Geometry: final body of the model. Coordinates: model frame, mm. Face numbers are marked on the shaded views. A direction names the side the tool comes from. Give positions to 0.01 mm unless a question says otherwise; leave off trailing zeros. Loops run counter-clockwise (first coordinate to the right, second up) from the corner with the lowest first, then second, coordinate; pieces in that order, holes last.
1. Access query for the marked faces 1 and 2. Directions: +Z, -Z, +X, -X, +Y, -Y. A direction counts if a zero-diameter tool reaches every point of the face in a straight line with its end or side. Return the directions, or none.
2. Section D-D, the plane z = -57.5. Output: boundary loops of the cut face in (x, y), then the cut area to 3 significant figures.
3. Material intervals for line 1 along Y through (x, z) = (2.25, -9); line 2 along Y through (x, z) = (2.25, -50); line 3 along Z through (x, y) = (2, 41.25), sorted ascending.
4. First-contact query: P1, Ø0.9, axis at x = 4.5, z = -26, coming from the +Y side; P2, Ø4, axis at y = 47, z = -23, coming from the -X side; P3, Ø6.5, axis at y = 47.5, z = -29.5, coming from the +X side; P4, Ø1.8, axis at y = 47, z = -37, coming from the +X side. Flat tips, straight axial feed; report the tip coordinate or a pass-through.
5. Section C-C, the plane z = -50. Output: boundary loops of the cut face in (x, y), then the cut area to 3 significant figures.
6. Section B-B, the plane y = 42. Output: boundary loops of the cut face in (x, z), then the cut area to 3 significant figures.
from build123d import *

# Parameters (mm, degrees)
SKETCH27_R          = 4
SKETCH27_R_2        = 2.5
BOSS_EXTRUDE1_DEPTH = 6
SKETCH33_R          = 4.99
CUT_EXTRUDE2_DEPTH  = 3
SKETCH34_W          = 20
SKETCH34_H          = 6
CUT_EXTRUDE3_DEPTH  = 3
CUT_EXTRUDE5_REACH  = 84.855
SKETCH36_R          = 1.5
FILLET3_R           = 2
FILLET4_R           = 10
CUT_EXTRUDE6_REACH  = 85.018
CHAMFER1_SIZE       = 1.5


with BuildPart() as part:
    # Sketch27 → Boss-Extrude1 (new body)
    with BuildSketch(Plane(origin=(0, 0, 0), x_dir=(0, 0, -1), z_dir=(1, 0, 0))):
        with BuildLine():
            Line((9, 50), (66, 50))
            Line((66, 50), (66, 45))
            Line((66, 45), (48.564398788, 34))
            Line((48.564398788, 34), (9, 34))
            ThreePointArc((9, 34), (1, 42), (9, 50))
        make_face()
        with Locations((9, 42)):
            Circle(SKETCH27_R, mode=Mode.SUBTRACT)
        with Locations((50, 42)):
            Circle(SKETCH27_R_2, mode=Mode.SUBTRACT)
    extrude(amount=BOSS_EXTRUDE1_DEPTH)

    # Sketch33 → Cut-Extrude2 (cut)
    with BuildSketch(Plane(origin=(6, 0, 0), x_dir=(0, 0, -1), z_dir=(1, 0, 0))):
        with Locations((9, 42)):
            Circle(SKETCH33_R)
    extrude(amount=-CUT_EXTRUDE2_DEPTH, mode=Mode.SUBTRACT)

    # Sketch34 → Cut-Extrude3 (cut)
    with BuildSketch(Plane(origin=(6, 0, 0), x_dir=(0, 0, -1), z_dir=(1, 0, 0))):
        with Locations((30, 47)):
            Rectangle(SKETCH34_W, SKETCH34_H)
    extrude(amount=-CUT_EXTRUDE3_DEPTH, mode=Mode.SUBTRACT)

    # Sketch36 → Cut-Extrude5 (cut, up to next)
    with BuildSketch(Plane(origin=(3, 0, 0), x_dir=(0, 0, -1), z_dir=(1, 0, 0)), mode=Mode.PRIVATE) as cut_extrude5_sk1:
        with Locations((23, 47)):
            Circle(SKETCH36_R)
    cut_extrude5_tool1 = extrude(cut_extrude5_sk1.sketch, amount=-CUT_EXTRUDE5_REACH, mode=Mode.PRIVATE) & part.part
    # Sketch36 → Cut-Extrude5 (cut, up to next)
    with BuildSketch(Plane(origin=(3, 0, 0), x_dir=(0, 0, -1), z_dir=(1, 0, 0)), mode=Mode.PRIVATE) as cut_extrude5_sk2:
        with Locations((37, 47)):
            Circle(SKETCH36_R)
    cut_extrude5_tool2 = extrude(cut_extrude5_sk2.sketch, amount=-CUT_EXTRUDE5_REACH, mode=Mode.PRIVATE) & part.part
    add(cut_extrude5_tool1.solids().sort_by_distance((3, 47, -23))[0], mode=Mode.SUBTRACT)
    add(cut_extrude5_tool2.solids().sort_by_distance((3, 47, -37))[0], mode=Mode.SUBTRACT)

    # Fillet3
    fillet3_edges = [part.edges().sort_by_distance(p)[0] for p in [
        (3, 50, -66),
        (3, 45, -66),
    ]]
    fillet(fillet3_edges, radius=FILLET3_R)

    # Fillet4
    fillet4_edges = [part.edges().sort_by_distance(p)[0] for p in [
        (3, 34, -48.564398788),
    ]]
    fillet(fillet4_edges, radius=FILLET4_R)

    # Sketch37 → Cut-Extrude6 (cut, up to next)
    with BuildSketch(Plane(origin=(6, 0, 0), x_dir=(0, 0, -1), z_dir=(1, 0, 0)), mode=Mode.PRIVATE) as cut_extrude6_sk1:
        with BuildLine():
            Line((20.313708499, 38), (42.254033308, 38))
            ThreePointArc((42.254033308, 38), (44.754033308, 37.682458366), (47.09526249, 36.75))
            ThreePointArc((47.09526249, 36.75), (50.17237218, 36.002476525), (53.201469536, 36.925495807))
            Line((53.201469536, 36.925495807), (53.201469536, 34))
            Line((53.201469536, 34), (9, 34))
            ThreePointArc((9, 34), (11.666666667, 34.457527667), (14.028314888, 35.777777778))
            ThreePointArc((14.028314888, 35.777777778), (16.980375166, 37.428090416), (20.313708499, 38))
        make_face()
    cut_extrude6_tool1 = extrude(cut_extrude6_sk1.sketch, amount=-CUT_EXTRUDE6_REACH, mode=Mode.PRIVATE) & part.part
    add(cut_extrude6_tool1.solids().sort_by_distance((6, 35.823598, -32.372789))[0], mode=Mode.SUBTRACT)

    # Chamfer1
    chamfer1_edges = [part.edges().sort_by_distance(p)[0] for p in [
        (0, 47, -21.5),
        (0, 47, -35.5),
    ]]
    chamfer(chamfer1_edges, length=CHAMFER1_SIZE - 0.0001)  # a hair under: the kernel refuses the full size


solid = part.part
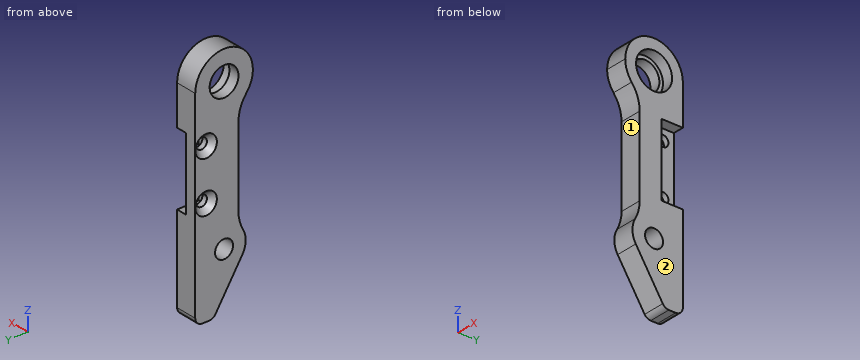
Answers below:
1. face 1: +X, -X, -Y
1. face 2: +Z, -Z, +X, +Y, -Y
2. outline: (0, 39.64) - (6, 39.64) - (6, 50) - (0, 50) - close
2. area: 62.2 mm2
3. line 1: y = 34 to 38, 46 to 50
3. line 2: y = 36 to 39.5, 44.5 to 50
3. line 3: z = -60.06 to -52.38, -47.62 to -12.93, -5.07 to -1.04
4. P1: stops at y = 44
4. P2: stops at x = 1
4. P3: stops at x = 3
4. P4: passes through
5. outline: (0, 36) - (6, 36) - (6, 39.5) - (0, 39.5) - close; (0, 44.5) - (6, 44.5) - (6, 50) - (0, 50) - close
5. area: 54.0 mm2
6. outline: (0, -61.24) - (6, -61.24) - (6, -52.5) - (0, -52.5) - close; (0, -47.5) - (6, -47.5) - (6, -13.99) - (3, -13.99) - (3, -13) - (0, -13) - close; (0, -5) - (3, -5) - (3, -4.01) - (6, -4.01) - (6, -1) - (0, -1) - close
6. area: 278 mm2
